Geometry: final body of the model. Coordinates: model frame, mm. Face numbers are marked on the shaded views. A direction names the side the tool comes from. Round coordinates to 2 decimals unless told otherwise and drop trailing zeros. Write each loop counter-clockwise with the first axis right and the second up, starting at its lowest first coordinate (ties: lowest second). Pieces come first, ordered by that corner, then holes. Notation, with made-up numbers: (-37, -1.75) -> (-1, -1.75) arc R21 ccw to (-1, 20.25) -> close; hole circle Ø5 at (56, 66). An arc over 180 degrees is marked (long way). One line per item, written item: value. Start each with the question number.
from build123d import *

# Parameters (mm, degrees)
F0_W     = 72.713092
F0_H     = 129.808232
F1_DEPTH = 63.5
F2_R     = 11.045044
F3_DEPTH = 129.809232
F4_W     = 76.8096
F4_H     = 25.091141
F5_DEPTH = 72.714092
F6_W     = 53.76672
F6_H     = 111.88598
F7_DEPTH = 63.501


with BuildPart() as f1:
    # F0 (on Top) → F1 (new body)
    with BuildSketch(Plane.XY):
        Rectangle(F0_W, F0_H)
    extrude(amount=F1_DEPTH)

    # F2 (on face) → F3 (cut, through all)
    with BuildSketch(Plane.XZ.offset(64.904116)):
        with Locations((0, 35.204399)):
            Circle(F2_R)
    extrude(amount=-F3_DEPTH, mode=Mode.SUBTRACT)

    # F4 (on face) → F5 (cut, through all)
    with BuildSketch(Plane.YZ.offset(36.356546)):
        with Locations((0, 51.334418)):
            Rectangle(F4_W, F4_H)
    extrude(amount=-F5_DEPTH, mode=Mode.SUBTRACT)

    # F6 (on Top) → F7 (cut, through all)
    with BuildSketch(Plane.XY):
        Rectangle(F6_W, F6_H)
    extrude(amount=F7_DEPTH, mode=Mode.SUBTRACT)


solid = f1.part
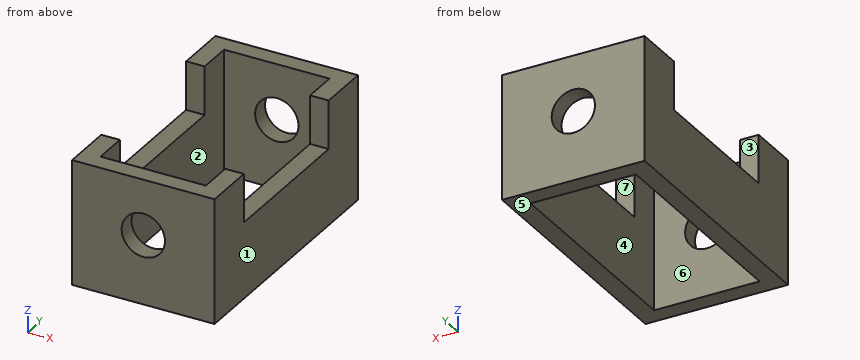
(1) Section query C-C (z = 12). Output: boundary loops of the cut face in (x, y).
(2) Set-up query: the marked faces 5, 6 and 7. Return all of +Z, -Z, +X, -X, +Y, -Y with unobstructed straight access to the full face (end or side cutting, diameter ignored); none if empty.
(3) Pin query (flat end, axial travel): pin 1 (10.5 mm diameter, centred on x = 32, y = 4.5, fed in from +Z). Return the tip coordinate at first contact, or that it passes through.
(4) Section query D-D (z = 49.5). Output: boundary loops of the cut face in (x, y), and give its area (3 significant figures).
(5) Line query: probe 1 along Z at (x, y) = (0, 59.5); probe 2 along Y at (x, z) = (-26.5, 8); probe 3 along X at (y, z) = (-53.5, 36). Output: solid intervals per line, ascending.
(6) Section query A-A (y = 53). Output: boundary loops of the cut face in (x, z).
(7) Section query B-B (x = 12.5). Output: boundary loops of the cut face in (y, z), and give its area (3 significant figures).
(8) Pull-direction query (X, two-part tool) for the marked faces 1, 2, 3 and 4; classes: pulls with the +X half, pulls with the -X half, needs draft (parallel to the pull), parting line crosses it, or undercut.
Results list:
1. outline: (-36.36, -64.9) -> (36.36, -64.9) -> (36.36, 64.9) -> (-36.36, 64.9) -> close; hole (-26.88, -55.94) -> (26.88, -55.94) -> (26.88, 55.94) -> (-26.88, 55.94) -> close
2. face 5: -Z, +X, -X, +Y, -Y
2. face 6: +Z, -Z
2. face 7: +Z, +X, -X
3. pin 1: stops at z = 38.79
4. outline: (-36.36, -64.9) -> (36.36, -64.9) -> (36.36, -38.4) -> (26.88, -38.4) -> (26.88, -55.94) -> (-26.88, -55.94) -> (-26.88, -38.4) -> (-36.36, -38.4) -> close; (-36.36, 38.4) -> (-26.88, 38.4) -> (-26.88, 55.94) -> (26.88, 55.94) -> (26.88, 38.4) -> (36.36, 38.4) -> (36.36, 64.9) -> (-36.36, 64.9) -> close
4. area: 1,970 mm^2
5. probe 1: z = 0 to 24.16, 46.25 to 63.5
5. probe 2: y = -64.9 to -55.94, 55.94 to 64.9
5. probe 3: x = -36.36 to -26.88, 26.88 to 36.36
6. outline: (-36.36, 0) -> (-26.88, 0) -> (-26.88, 63.5) -> (-36.36, 63.5) -> close; (26.88, 0) -> (36.36, 0) -> (36.36, 63.5) -> (26.88, 63.5) -> close
7. outline: (-64.9, 0) -> (-55.94, 0) -> (-55.94, 63.5) -> (-64.9, 63.5) -> close; (55.94, 0) -> (64.9, 0) -> (64.9, 63.5) -> (55.94, 63.5) -> close
7. area: 1,140 mm^2
8. face 1: pulls with the +X half
8. face 2: undercut
8. face 3: needs draft
8. face 4: undercut
